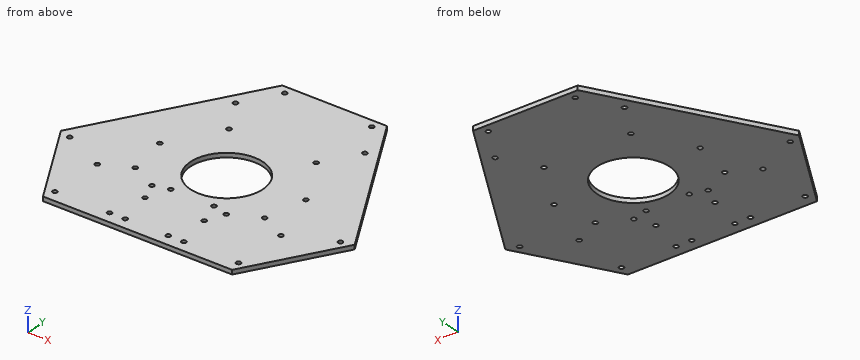
from build123d import *

# Parameters (mm, degrees)
SKETCH_1_R          = 1.6
SKETCH_1_R_2        = 25
EXTRUDE_1_DEPTH     = 3
SKETCH_2_R          = 1.6
CUT_EXTRUDE_1_DEPTH = 4


with BuildPart() as part:
    # ｽｹｯﾁ1 → ﾎﾞｽ - 押し出し1 (new body)
    with BuildSketch(Plane.XY):
        Polygon((-36.39879245, 96.955442142), (36.39879245, 96.955442142), (102.165272155, -16.955442142), (65.766479705, -80), (-65.766479705, -80), (-102.165272155, -16.955442142), align=None)
        with Locations((30.25, 91.195498156)):
            Circle(SKETCH_1_R, mode=Mode.SUBTRACT)
        with Locations((30.25, 41.195498156)):
            Circle(SKETCH_1_R, mode=Mode.SUBTRACT)
        with Locations((-30.25, 41.195498156)):
            Circle(SKETCH_1_R, mode=Mode.SUBTRACT)
        with Locations((-30.25, 91.195498156)):
            Circle(SKETCH_1_R, mode=Mode.SUBTRACT)
        with Locations((63.852618114, -71.795017542)):
            Circle(SKETCH_1_R, mode=Mode.SUBTRACT)
        with Locations((94.102618114, -19.400480613)):
            Circle(SKETCH_1_R, mode=Mode.SUBTRACT)
        with Locations((50.801347925, 5.599519387)):
            Circle(SKETCH_1_R, mode=Mode.SUBTRACT)
        with Locations((20.551347925, -46.795017542)):
            Circle(SKETCH_1_R, mode=Mode.SUBTRACT)
        with Locations((-94.102618114, -19.400480613)):
            Circle(SKETCH_1_R, mode=Mode.SUBTRACT)
        with Locations((-63.852618114, -71.795017542)):
            Circle(SKETCH_1_R, mode=Mode.SUBTRACT)
        with Locations((-20.551347925, -46.795017542)):
            Circle(SKETCH_1_R, mode=Mode.SUBTRACT)
        with Locations((-50.801347925, 5.599519387)):
            Circle(SKETCH_1_R, mode=Mode.SUBTRACT)
        Circle(SKETCH_1_R_2, mode=Mode.SUBTRACT)
    extrude(amount=EXTRUDE_1_DEPTH)

    # ｽｹｯﾁ2 → ｶｯﾄ - 押し出し1 (cut, through all)
    with BuildSketch(Plane(origin=(0, 0, 0), x_dir=(-1, 0, 0), z_dir=(0, 0, -1))):
        with Locations((-63.852618114, -33.795017542)):
            Circle(SKETCH_2_R)
        with Locations((-25.852618114, -33.795017542)):
            Circle(SKETCH_2_R)
        with Locations((-25.852618114, -71.795017542)):
            Circle(SKETCH_2_R)
        with Locations((-63.852618114, -71.795017542)):
            Circle(SKETCH_2_R)
        with Locations((15, -30.795017542)):
            Circle(SKETCH_2_R)
        with Locations((-15, -30.795017542)):
            Circle(SKETCH_2_R)
        with Locations((-15, -71.795017542)):
            Circle(SKETCH_2_R)
        with Locations((15, -71.795017542)):
            Circle(SKETCH_2_R)
        with Locations((45, 66)):
            Circle(SKETCH_2_R)
        with Locations((-45, 66)):
            Circle(SKETCH_2_R)
        with Locations((-45, -24)):
            Circle(SKETCH_2_R)
        with Locations((45, -24)):
            Circle(SKETCH_2_R)
        with Locations((63.852618114, -71.795017542)):
            Circle(SKETCH_2_R)
        with Locations((25.852618114, -71.795017542)):
            Circle(SKETCH_2_R)
        with Locations((25.852618114, -33.795017542)):
            Circle(SKETCH_2_R)
        with Locations((63.852618114, -33.795017542)):
            Circle(SKETCH_2_R)
    extrude(amount=-CUT_EXTRUDE_1_DEPTH, mode=Mode.SUBTRACT)


solid = part.part
Work out the finished part from the listing and answer in its coordinate system (mm). Coordinates: 2 decimals unless noted, no trailing zeros. Loops run counter-clockwise (first coordinate to the right, second up) from the corner with the lowest first, then second, coordinate; pieces in that order, holes last. Notation, with made-up numbers: (10.5, 31) -> (44.5, 31) arc R25 cw to (44.5, 64) -> close; hole circle Ø3 at (-5, 35). An arc over 180 degrees is marked (long way). Answer as CSV lines item,"result".
1) The part is cut by section D-D (x = -80). Give the vertices of the cut face in (y, z).
A:
outline,"(-55.35, 0) -> (21.44, 0) -> (21.44, 3) -> (-55.35, 3) -> close"
2) The part is cut by section B-B (y = 0). Give the vertices of the cut face in (x, z).
A:
outline,"(-92.38, 0) -> (-25, 0) -> (-25, 3) -> (-92.38, 3) -> close; (25, 0) -> (92.38, 0) -> (92.38, 3) -> (25, 3) -> close"
3) Flat-ended cylindrical pins translate along their axes: pin 1 (2.5 mm diameter, centred on x = 15, y = -71.8, fed in from -Z); pin 2 (1.5 mm diameter, centred on y = 65.5, z = 2, fed in from +X); pin 3 (1 mm diameter, centred on y = 1.5, z = 1.5, fed in from -X). Find the tip coordinate at first contact, or state that the pin passes through.
A:
pin 1,"passes through"
pin 2,"stops at x = 54.99"
pin 3,"stops at x = -91.8"
4) Straight lines are drawn through the part: probe 1 along Y at (x, z) = (63.5, 2.1); probe 2 along Y at (x, z) = (-15, 1.75); probe 3 along X at (y, z) = (-23, 2.05). For each, find the intervals that lie inside material, in ascending order.
A:
probe 1,"y = -80 to -73.36, -70.23 to -35.36, -32.23 to 50.01"
probe 2,"y = -80 to -73.4, -70.2 to -32.4, -29.2 to -20, 20 to 96.96"
probe 3,"x = -98.68 to -46.25, -43.75 to -9.8, 9.8 to 43.75, 46.25 to 98.68"
5) The part is cut by section A-A (x = 0). Give the vertices of the cut face in (y, z), and give its area (3 significant figures).
A:
outline,"(-80, 0) -> (-25, 0) -> (-25, 3) -> (-80, 3) -> close; (25, 0) -> (96.96, 0) -> (96.96, 3) -> (25, 3) -> close"
area,"381 mm²"
6) The part is cut by section C-C (z = 2.05). State how many separate pieces and enclosed holes the cut face has, and give its area (3 significant figures).
A:
separate pieces,"1"
enclosed holes,"27"
area,"24,200 mm²"
